Build history of the part. All positions in model axes, mm. Face numbers are marked on the shaded views. A direction names the side the tool comes from. Give positions to 0.01 mm unless a question says otherwise; leave off trailing zeros. Write each loop counter-clockwise with the first axis right and the second up, starting at its lowest first coordinate (ties: lowest second). Pieces come first, ordered by that corner, then holes. Notation, with made-up numbers: (77, -9.5) -> (124, -9.5) arc R3 ccw to (124, -5.5) -> close; hole circle Ø1 at (-9.75, 6.25). An arc over 180 degrees is marked (long way). Put each result on its own line as item: value. Start each with the question number.
Item 1: Drill centre lines: line 1 along Z through (x, y) = (0, -8); line 2 along Z through (x, y) = (-16.5, -20.5); line 3 along X through (y, z) = (-6.25, 0). Where is each one in solid material? Low to high.
Item 2: Slice it at B-B, the plane z = 0. List the corners of the cut face in (x, y), plus the area to 3 significant figures.
Item 3: Slice it at C-C, the plane z = -20. List the corners of the cut face in (x, y).
Item 4: Two-plate mould, pull along X, no slides. Class the marked faces 4, 5, 6 and 7: pulls with the +X half, pulls with the -X half, needs draft (parallel to the pull), parting line crosses it, or undercut.
Item 5: Slice it at A-A, the plane x = 0. List the corners of the cut face in (y, z).
Item 6: Flat gauge pins, fed straight in: pin 1 Ø2 at (x, y) = (-13, -15) entering from -Z; pin 2 Ø12 at (x, y) = (11.5, -26) entering from +Z; pin 3 Ø1.5 at (x, y) = (-13, -24.5) entering from +Z. Where does each tip first touch, or does it go through?
Item 7: Tool access for the marked faces 1, 2 and 3: list every direction of +Z, -Z, +X, -X, +Y, -Y with a clear straight run to the whole face (end or side of a thin tool).
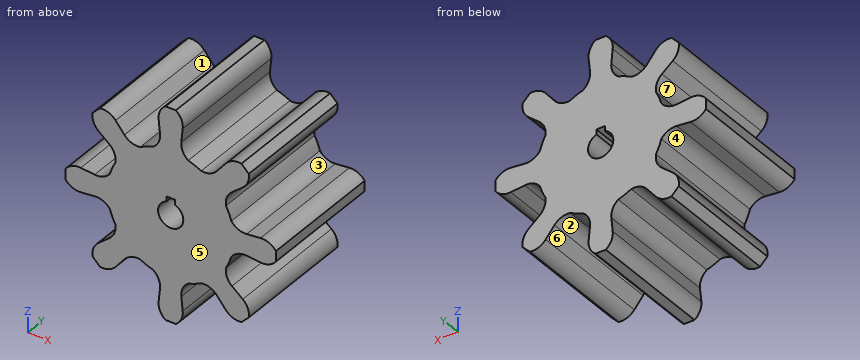
```python
from build123d import *

# Parameters (mm, degrees)
F1_DEPTH = 30
F3_DEPTH = 30.001


with BuildPart() as f1:
    # F0 (on Front) → F1 (new body)
    with BuildSketch(Plane.XZ):
        with BuildLine():
            ThreePointArc((-14.555619, 10.982389), (-13.34453, 9.30297), (-13.135405, 7.243005))
            ThreePointArc((-13.135405, 7.243005), (-13.858193, 5.740251), (-14.409712, 4.166556))
            ThreePointArc((-14.409712, 4.166556), (-16.0142, 2.857814), (-18.058099, 2.526655))
            Line((-18.058099, 2.526655), (-21.351614, 2.861007))
            ThreePointArc((-21.351614, 2.861007), (-23.395512, 2.529847), (-25, 1.221105))
            Line((-25, 1.221105), (-25, -1.221105))
            ThreePointArc((-25, -1.221105), (-23.395512, -2.529847), (-21.351614, -2.861007))
            Line((-21.351614, -2.861007), (-18.058099, -2.526655))
            ThreePointArc((-18.058099, -2.526655), (-16.0142, -2.857814), (-14.409712, -4.166556))
            ThreePointArc((-14.409712, -4.166556), (-13.858193, -5.740251), (-13.135405, -7.243005))
            ThreePointArc((-13.135405, -7.243005), (-13.34453, -9.30297), (-14.555619, -10.982389))
            Line((-14.555619, -10.982389), (-17.120908, -13.074834))
            ThreePointArc((-17.120908, -13.074834), (-18.331997, -14.754253), (-18.541121, -16.814218))
            Line((-18.541121, -16.814218), (-16.814218, -18.541121))
            ThreePointArc((-16.814218, -18.541121), (-14.754253, -18.331997), (-13.074834, -17.120908))
            Line((-13.074834, -17.120908), (-10.982389, -14.555619))
            ThreePointArc((-10.982389, -14.555619), (-9.30297, -13.34453), (-7.243005, -13.135405))
            ThreePointArc((-7.243005, -13.135405), (-5.740251, -13.858193), (-4.166556, -14.409712))
            ThreePointArc((-4.166556, -14.409712), (-2.857814, -16.0142), (-2.526655, -18.058099))
            Line((-2.526655, -18.058099), (-2.861007, -21.351614))
            ThreePointArc((-2.861007, -21.351614), (-2.529847, -23.395512), (-1.221105, -25))
            Line((-1.221105, -25), (1.221105, -25))
            ThreePointArc((1.221105, -25), (2.529847, -23.395512), (2.861007, -21.351614))
            Line((2.861007, -21.351614), (2.526655, -18.058099))
            ThreePointArc((2.526655, -18.058099), (2.857814, -16.0142), (4.166556, -14.409712))
            ThreePointArc((4.166556, -14.409712), (5.740251, -13.858193), (7.243005, -13.135405))
            ThreePointArc((7.243005, -13.135405), (9.30297, -13.34453), (10.982389, -14.555619))
            Line((10.982389, -14.555619), (13.074834, -17.120908))
            ThreePointArc((13.074834, -17.120908), (14.754253, -18.331997), (16.814218, -18.541121))
            Line((16.814218, -18.541121), (18.541121, -16.814218))
            ThreePointArc((18.541121, -16.814218), (18.331997, -14.754253), (17.120908, -13.074834))
            Line((17.120908, -13.074834), (14.555619, -10.982389))
            ThreePointArc((14.555619, -10.982389), (13.34453, -9.30297), (13.135405, -7.243005))
            ThreePointArc((13.135405, -7.243005), (13.858193, -5.740251), (14.409712, -4.166556))
            ThreePointArc((14.409712, -4.166556), (16.0142, -2.857814), (18.058099, -2.526655))
            Line((18.058099, -2.526655), (21.351614, -2.861007))
            ThreePointArc((21.351614, -2.861007), (23.395512, -2.529847), (25, -1.221105))
            Line((25, -1.221105), (25, 1.221105))
            ThreePointArc((25, 1.221105), (23.395512, 2.529847), (21.351614, 2.861007))
            Line((21.351614, 2.861007), (18.058099, 2.526655))
            ThreePointArc((18.058099, 2.526655), (16.0142, 2.857814), (14.409712, 4.166556))
            ThreePointArc((14.409712, 4.166556), (13.858193, 5.740251), (13.135405, 7.243005))
            ThreePointArc((13.135405, 7.243005), (13.34453, 9.30297), (14.555619, 10.982389))
            Line((14.555619, 10.982389), (17.120908, 13.074834))
            ThreePointArc((17.120908, 13.074834), (18.331997, 14.754253), (18.541121, 16.814218))
            Line((18.541121, 16.814218), (16.814218, 18.541121))
            ThreePointArc((16.814218, 18.541121), (14.754253, 18.331997), (13.074834, 17.120908))
            Line((13.074834, 17.120908), (10.982389, 14.555619))
            ThreePointArc((10.982389, 14.555619), (9.30297, 13.34453), (7.243005, 13.135405))
            ThreePointArc((7.243005, 13.135405), (5.740251, 13.858193), (4.166556, 14.409712))
            ThreePointArc((4.166556, 14.409712), (2.857814, 16.0142), (2.526655, 18.058099))
            Line((2.526655, 18.058099), (2.861007, 21.351614))
            ThreePointArc((2.861007, 21.351614), (2.529847, 23.395512), (1.221105, 25))
            Line((1.221105, 25), (-1.221105, 25))
            ThreePointArc((-1.221105, 25), (-2.529847, 23.395512), (-2.861007, 21.351614))
            Line((-2.861007, 21.351614), (-2.526655, 18.058099))
            ThreePointArc((-2.526655, 18.058099), (-2.857814, 16.0142), (-4.166556, 14.409712))
            ThreePointArc((-4.166556, 14.409712), (-5.740251, 13.858193), (-7.243005, 13.135405))
            ThreePointArc((-7.243005, 13.135405), (-9.30297, 13.34453), (-10.982389, 14.555619))
            Line((-10.982389, 14.555619), (-13.074834, 17.120908))
            ThreePointArc((-13.074834, 17.120908), (-14.754253, 18.331997), (-16.814218, 18.541121))
            Line((-16.814218, 18.541121), (-18.541121, 16.814218))
            ThreePointArc((-18.541121, 16.814218), (-18.331997, 14.754253), (-17.120908, 13.074834))
            Line((-17.120908, 13.074834), (-14.555619, 10.982389))
        make_face()
    extrude(amount=F1_DEPTH)

    # F2 (on face) → F3 (cut, through all)
    with BuildSketch(Plane.XZ.offset(30)):
        with BuildLine():
            Line((-1, 4), (-1, 2.828427))
            ThreePointArc((-1, 2.828427), (0, -3), (1, 2.828427))
            Line((1, 2.828427), (1, 4))
            Line((1, 4), (-1, 4))
        make_face()
    extrude(amount=-F3_DEPTH, mode=Mode.SUBTRACT)


solid = f1.part
```
Values follow:
1. line 1: -25 to -3, 4 to 25
1. line 2: -18.58 to -12.57, -2.68 to 2.68, 12.57 to 18.58
1. line 3: -25 to -3, 3 to 25
2. outline: (-25, -30) -> (-3, -30) -> (-3, 0) -> (-25, 0) -> close; (3, -30) -> (25, -30) -> (25, 0) -> (3, 0) -> close
2. area: 1,320 mm2
3. outline: (-2.72, -30) -> (2.72, -30) -> (2.72, 0) -> (-2.72, 0) -> close
4. face 4: undercut
4. face 5: needs draft
4. face 6: undercut
4. face 7: pulls with the -X half
5. outline: (-30, -25) -> (0, -25) -> (0, -3) -> (-30, -3) -> close; (-30, 4) -> (0, 4) -> (0, 25) -> (-30, 25) -> close
6. pin 1: z = -17.95
6. pin 2: z = 18.59
6. pin 3: z = 17.77
7. face 1: +Z, +Y, -Y
7. face 2: -Z, +Y, -Y
7. face 3: +Y, -Y
